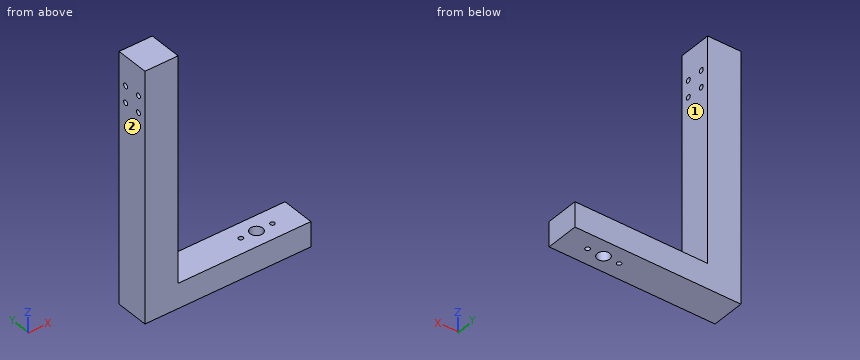
```python
from build123d import *

# Parameters (mm, degrees)
BOSS_EXTRUDE2_DEPTH = 40
SKETCH3_R           = 3
CUT_EXTRUDE1_DEPTH  = 265.256065707
SKETCH4_R           = 3
CUT_EXTRUDE2_DEPTH  = 40
SKETCH5_R           = 7.5
CUT_EXTRUDE3_DEPTH  = 40
SKETCH6_R           = 2.735775354
CUT_EXTRUDE4_DEPTH  = 40


with BuildPart() as part:
    # Sketch2 → Boss-Extrude2 (new body)
    with BuildSketch(Plane(origin=(0, 0, 0), x_dir=(1, 0, 0), z_dir=(0, 1, 0))):
        Polygon((-59.708737864, 220.339805825), (140.291262136, 220.339805825), (140.291262136, 190.339805825), (-19.708737864, 190.339805825), (-19.708737864, -79.660194175), (-59.708737864, -79.660194175), align=None)
    extrude(amount=BOSS_EXTRUDE2_DEPTH)

    # Sketch3 → Cut-Extrude1 (cut, through all)
    with BuildSketch(Plane(origin=(0, 0, 0), x_dir=(0, 0, -1), z_dir=(1, 0, 0))):
        with Locations((-24.660194175, 30)):
            Circle(SKETCH3_R)
        with Locations((-44.660194175, 30)):
            Circle(SKETCH3_R)
    extrude(amount=-CUT_EXTRUDE1_DEPTH, mode=Mode.SUBTRACT)

    # Sketch4 → Cut-Extrude2 (cut)
    with BuildSketch(Plane(origin=(-19.708737864, 0, 0), x_dir=(0, 0, -1), z_dir=(1, 0, 0))):
        with Locations((-44.660194175, 10)):
            Circle(SKETCH4_R)
        with Locations((-24.660194175, 10)):
            Circle(SKETCH4_R)
    extrude(amount=-CUT_EXTRUDE2_DEPTH, mode=Mode.SUBTRACT)

    # Sketch5 → Cut-Extrude3 (cut)
    with BuildSketch(Plane(origin=(0, 0, -220.339805825), x_dir=(-1, 0, 0), z_dir=(0, 0, -1))):
        with Locations((-90.291262136, 20)):
            Circle(SKETCH5_R)
    extrude(amount=-CUT_EXTRUDE3_DEPTH, mode=Mode.SUBTRACT)

    # Sketch6 → Cut-Extrude4 (cut)
    with BuildSketch(Plane(origin=(0, 0, -220.339805825), x_dir=(-1, 0, 0), z_dir=(0, 0, -1))):
        with Locations((-109.465398349, 20)):
            Circle(SKETCH6_R)
        with Locations((-71.49377823, 20)):
            Circle(SKETCH6_R)
    extrude(amount=-CUT_EXTRUDE4_DEPTH, mode=Mode.SUBTRACT)


solid = part.part
```
Work out the finished part from the listing and answer in its coordinate system (mm). Face numbers are marked on the shaded views. A direction names the side the tool comes from. Coordinates: 2 decimals unless noted, no trailing zeros. Write each loop counter-clockwise with the first axis right and the second up, starting at its lowest first coordinate (ties: lowest second). Pieces come first, ordered by that corner, then holes.
Q1. A cutting plane is placed at B-B, the plane x = 42. Give the vertices of the cut face in (y, z).
Q2. Find the intervals of material crossed by line 1 (Z direction, x = -42.5, y = 30.5); line 2 (X direction, y = 17.5, z = -3.5); line 3 (Z direction, x = 72, y = 35), in increasing order.
Q3. Each of these flat-tipped pins is pushed along its axis until it touches: pin 1 Ø12 at (y, z) = (28.5, -5.5) entering from +X; pin 2 Ø19.5 at (x, y) = (90.29, 20) entering from -Z; pin 3 Ø6.5 at (x, y) = (71.49, 20) entering from +Z. Where does it stop, or does it pass through?
Q4. A cutting plane is placed at A-A, the plane z = -77. Give the vertices of the cut face in (x, y).
Q5. Which of the six approach directions +Z, -Z, +X, -X, +Y, -Y give full straight-line access (tool end or side, diameter ignored) to the marked faces 1 and 2?
Findings below:
1. outline: (0, -220.34) - (40, -220.34) - (40, -190.34) - (0, -190.34) - close
2. line 1: z = -220.34 to 21.7, 27.62 to 41.7, 47.62 to 79.66
2. line 2: x = -59.71 to -19.71
2. line 3: z = -220.34 to -190.34
3. pin 1: stops at x = -19.71
3. pin 2: stops at z = -220.34
3. pin 3: stops at z = -190.34
4. outline: (-59.71, 0) - (-19.71, 0) - (-19.71, 40) - (-59.71, 40) - close
5. face 1: +Z, +X, +Y, -Y
5. face 2: +Z, -Z, -X, +Y, -Y
